Input: dimensioned drawing with shaded views. Units: mm. Origin: part minimum x, y, z. A direction names the side the tool comes from. Round coordinates to 2 decimals unless told otherwise and drop trailing zeros. Loops run counter-clockwise (first coordinate to the right, second up) from the corner with the lowest first, then second, coordinate; pieces in that order, holes last. Notation, with made-up numbers: (52, 15.25) - (98, 15.25) arc R13 cw to (98, 27.25) - close; hole circle Ø9 at (84, -21). An arc over 180 degrees is marked (long way). Answer as a JSON object with one key per item and string values. Group by question number.
Item 1: Section B-B (x = 88.9). Count the separate pieces of the cut face and the enclosed holes in it, plus the area to 3 significant figures.
Item 2: Line query: line 1 (Z direction, x = 88.9, y = 10.25); line 2 (Y direction, x = 157.5, z = 109); line 3 (X direction, y = 6.75, z = 99.5) (1 decimal). Output: solid intervals per line, ascending.
Item 3: Reachability of the marked faces 1 and 2 from +Z, -Z, +X, -X, +Y, -Y: full face, straight path, thin tool, end or side. Return the list, or none.
Item 4: First-contact query: pin 1 (6 mm diameter, centred on x = 147, y = 6, fed in from +Z); pin 2 (1 mm diameter, centred on x = 45, y = 8.5, fed in from -Z); pin 3 (15 mm diameter, centred on x = 33.91, z = 57.15, fed in from -Y); pin 4 (1.5 mm diameter, centred on y = 10, z = 66, fed in from +X). Flat tips, straight axial feed; report the tip coordinate or a pass-through.
Item 5: Section C-C (x = 30). Return the cut outline in (y, z).
Item 6: Draft query along X for the marked faces 3 and 4. Return one class per face: released by +X, released by -X, zero draft, split by the parting line, or undercut.
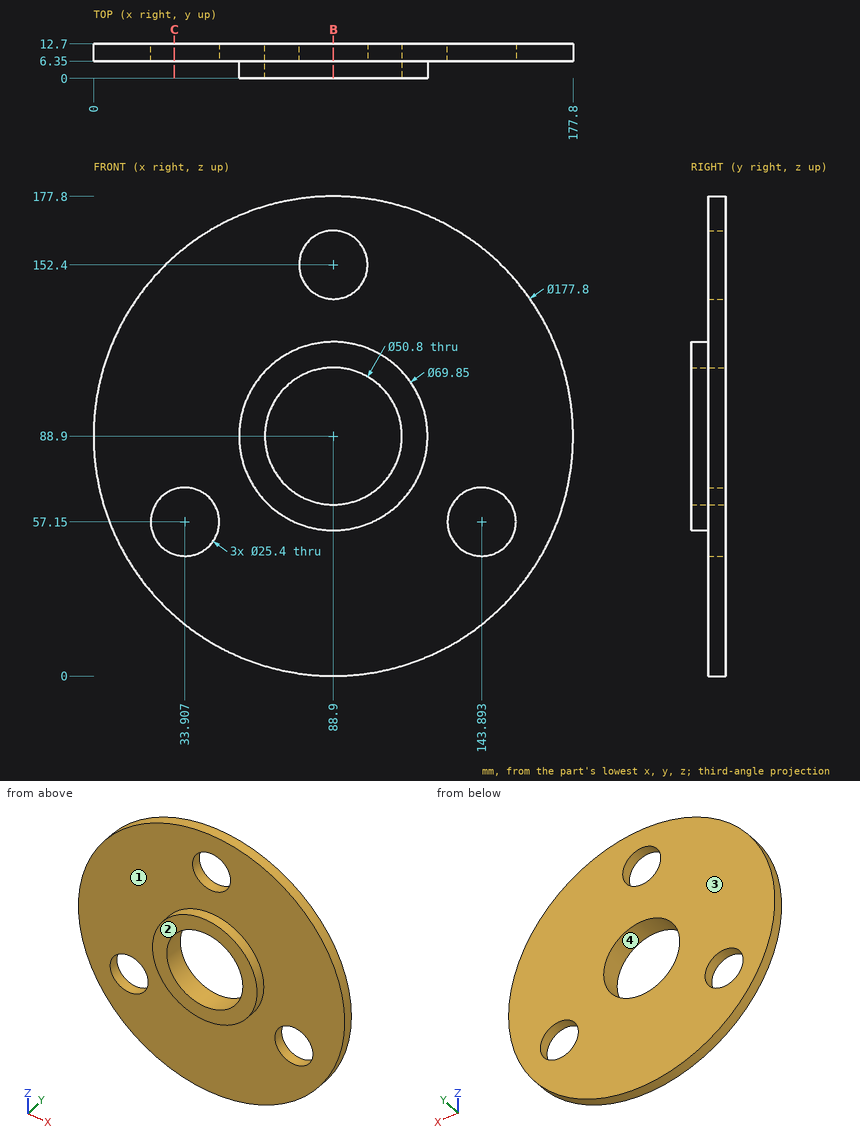
Values:
{
 "1": {"separate pieces": "3", "enclosed holes": "0", "area": "766 mm^2"},
 "2": {"line 1": "z = 0 to 63.5, 114.3 to 139.7, 165.1 to 177.8", "line 2": "y = 6.35 to 12.7", "line 3": "x = 0.6 to 65.8, 112 to 177.2"},
 "3": {"face 1": "-Y", "face 2": "+Z, -Z, +X, -X, -Y"},
 "4": {"pin 1": "stops at z = 158.65", "pin 2": "stops at z = 11.31", "pin 3": "passes through", "pin 4": "stops at x = 175"},
 "5": {"outline": "(6.35, 22.31) - (12.7, 22.31) - (12.7, 45.07) - (6.35, 45.07) - close; (6.35, 69.23) - (12.7, 69.23) - (12.7, 155.49) - (6.35, 155.49) - close"},
 "6": {"face 3": "zero draft", "face 4": "undercut"}
}
